CAD build for the part. Positions are in the model's coordinates, mm. Face numbers are marked on the shaded views. A direction names the side the tool comes from. Round coordinates to 2 decimals unless told otherwise and drop trailing zeros. Order: outer loops, then holes, each group sorted by start corner. A loop starts at its lowest first (then second) coordinate and runs counter-clockwise, first axis right, second up. Notation, with made-up numbers: M -4.5,9.25 L 52.5,9.25 A32 ccw 52.5,36.25 Z; hole C 47,27 d10. An arc over 180 degrees is marked long. Answer as a JSON object with one key per item and string values.
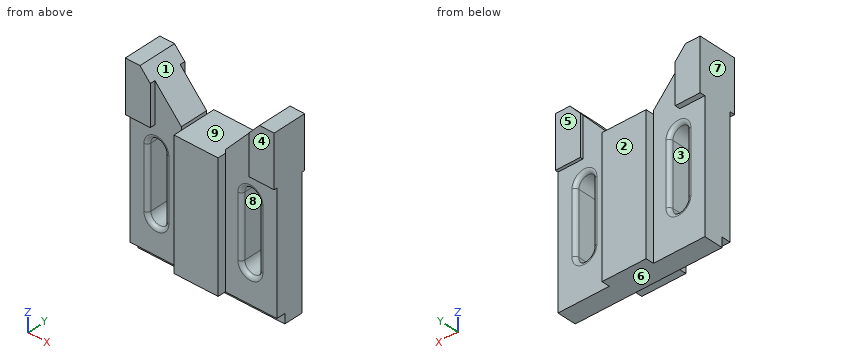
```python
from build123d import *

# Parameters (mm, degrees)
F1_DEPTH  = 15
F3_W      = 11.5
F3_H      = 6.5
F4_DEPTH  = 100
F6_DEPTH  = 5.5
F8_DEPTH  = 3.5
F10_DEPTH = 5.5
F12_DEPTH = 3.5
F14_DEPTH = 25
F15_R     = 2.5
F16_W     = 20.5905072875
F16_H     = 35
F16_W_2   = 2
F17_DEPTH = 17


with BuildPart() as f1:
    # F0 (on Front) → F1 (new body, symmetric)
    with BuildSketch(Plane.XZ):
        Polygon((0, 122), (0, 0), (100, 0), (100, 122), (90, 122), (65, 94.2346871293), (65, 92), (35, 92), (35, 94.2346871293), (10, 122), align=None)
    extrude(amount=F1_DEPTH, both=True)

    # F3 (on face) → F4 (cut)
    with BuildSketch(Plane(origin=(0, 0, 0), x_dir=(0, -1, 0), z_dir=(-1, 0, 0))):
        with Locations((9.25, 3.25)):
            Rectangle(F3_W, F3_H)
    extrude(amount=-F4_DEPTH, mode=Mode.SUBTRACT)

    # F5 (on face) → F6 (cut)
    with BuildSketch(Plane.XZ.offset(15)):
        Polygon((17, 87), (0, 87), (0, 6.5), (35, 6.5), (35, 92), (35, 94.2346871293), (17, 114.2257123962), align=None)
        Polygon((65, 94.2346871293), (65, 92), (65, 6.5), (100, 6.5), (100, 87), (83, 87), (83, 114.2257123962), align=None)
    extrude(amount=-F6_DEPTH, mode=Mode.SUBTRACT)

    # F7 (on face) → F8 (cut)
    with BuildSketch(Plane.XZ.offset(15)):
        Polygon((100, 122), (90, 122), (83, 114.2257123962), (83, 87), (100, 87), align=None)
    extrude(amount=-F8_DEPTH, mode=Mode.SUBTRACT)

    # F9 (on face) → F10 (cut)
    with BuildSketch(Plane(origin=(0, 15, 0), x_dir=(-1, 0, 0), z_dir=(0, 1, 0))):
        Polygon((-17, 87), (-17, 114.2257123962), (-35, 94.2346871293), (-35, 92), (-35, 0), (0, 0), (0, 87), align=None)
        Polygon((-65, 92), (-65, 94.2346871293), (-83, 114.2257123962), (-83, 87), (-100, 87), (-100, 0), (-65, 0), align=None)
    extrude(amount=-F10_DEPTH, mode=Mode.SUBTRACT)

    # F11 (on face) → F12 (cut)
    with BuildSketch(Plane(origin=(0, 15, 0), x_dir=(-1, 0, 0), z_dir=(0, 1, 0))):
        Polygon((-90, 122), (-100, 122), (-100, 87), (-83, 87), (-83, 114.2257123962), align=None)
    extrude(amount=-F12_DEPTH, mode=Mode.SUBTRACT)

    # F13 (on face) → F14 (cut)
    with BuildSketch(Plane.XZ.offset(15)):
        with BuildLine():
            Line((24, 30), (24, 72))
            ThreePointArc((24, 72), (18, 78), (12, 72))
            Line((12, 72), (12, 30))
            ThreePointArc((12, 30), (18, 24), (24, 30))
        make_face()
        with BuildLine():
            ThreePointArc((88, 72), (82, 78), (76, 72))
            Line((76, 72), (76, 30))
            ThreePointArc((76, 30), (82, 24), (88, 30))
            Line((88, 30), (88, 72))
        make_face()
    extrude(amount=-F14_DEPTH, mode=Mode.SUBTRACT)

    # F15
    f15_edges = [f1.edges().sort_by_distance(p)[0] for p in [
        (76, 9.5, 51),
        (24, 9.5, 51),
        (12, -9.5, 51),
        (76, -9.5, 51),
    ]]
    fillet(f15_edges, radius=F15_R)

    # F16 (on face) → F17 (cut)
    with BuildSketch(Plane(origin=(0, 0, 0), x_dir=(0, -1, 0), z_dir=(-1, 0, 0))):
        with Locations((-25.2952536438, 104.5)):
            Rectangle(F16_W, F16_H)
        with Locations((25.2952536438, 104.5)):
            Rectangle(F16_W, F16_H)
        with Locations((-14, 104.5)):
            Rectangle(F16_W_2, F16_H)
        with Locations((14, 104.5)):
            Rectangle(F16_W_2, F16_H)
    extrude(amount=-F17_DEPTH, mode=Mode.SUBTRACT)


solid = f1.part
```
Item 1: Saw through at D-D on z = 109. List the corners of the cut face in (x, y), and give its area (3 significant figures).
Worked answers:
{"outline": "M 0,-13 L 17,-13 L 17,-9.5 L 21.71,-9.5 L 21.71,9.5 L 17,9.5 L 17,13 L 0,13 Z; M 78.29,-9.5 L 83,-9.5 L 83,-11.5 L 100,-11.5 L 100,11.5 L 83,11.5 L 83,9.5 L 78.29,9.5 Z", "area": "1,010 mm2"}
Item 2: Saw through at A-A on y = 3.75. List the corners of the cut face in (x, z), and give its area (3 significant figures).
Worked answers:
{"outline": "M 0,0 L 100,0 L 100,122 L 90,122 L 65,94.23 L 65,92 L 35,92 L 35,94.23 L 10,122 L 0,122 Z; hole M 12,30 A6 ccw 24,30 L 24,72 A6 ccw 12,72 Z; hole M 76,30 A6 ccw 88,30 L 88,72 A6 ccw 76,72 Z", "area": "9,370 mm2"}
Item 3: Saw through at C-C on x = 49. List the corners of the cut face in (y, z).
Worked answers:
{"outline": "M -15,6.5 L -3.5,6.5 L -3.5,0 L 15,0 L 15,92 L -15,92 Z"}
Item 4: Saw through at B-B on z = 64. List the corners of the cut face in (x, y).
Worked answers:
{"outline": "M 0,-9.5 L 9.5,-9.5 A2.5 ccw 12,-7 L 12,7 A2.5 ccw 9.5,9.5 L 0,9.5 Z; M 24,-7 A2.5 ccw 26.5,-9.5 L 35,-9.5 L 35,-15 L 65,-15 L 65,-9.5 L 73.5,-9.5 A2.5 ccw 76,-7 L 76,7 A2.5 ccw 73.5,9.5 L 65,9.5 L 65,15 L 35,15 L 35,9.5 L 26.5,9.5 A2.5 ccw 24,7 Z; M 88,-7 A2.5 ccw 90.5,-9.5 L 100,-9.5 L 100,9.5 L 90.5,9.5 A2.5 ccw 88,7 Z"}
Item 5: 3-axis set-ups, long thin cutter, end or side, ignore diameter. For the marked faces 1, 2, 3, 4 and 5: which of +Z, -Z, +X, -X, +Y, -Y reach the whole face in a straight line?
Worked answers:
{"face 1": "+Z, +Y, -Y", "face 2": "+Z, -Z, +X, -X, +Y", "face 3": "+Y, -Y", "face 4": "+Z, -Z, +X, -Y", "face 5": "+Z, -Z, +X, +Y"}
Item 6: Wall check: line 1 along X through (y, z) = (2.5, 30); line 2 along X through (y, z) = (-12.5, 76); line 3 along Y through (x, z) = (7, 106). Give the ranges that are in metal, low to high. Write a range as [from, to].
Worked answers:
{"line 1": "x = [0, 12], [24, 76], [88, 100]", "line 2": "x = [35, 65]", "line 3": "y = [-13, 13]"}
Item 7: Drop flat-ended pins along their axis: pin 1 Ø3 at (y, z) = (-12.5, 64) entering from -X; pin 2 Ø17.5 at (x, z) = (85.5, 52) entering from +Y; pin 3 Ø3 at (x, y) = (38, 11) entering from +Z. Give the stop position or say it passes through.
Worked answers:
{"pin 1": "stops at x = 35", "pin 2": "stops at y = 9.5", "pin 3": "stops at z = 92"}
Item 8: Two-plate mould, pull along X, no slides. Class the marked faces 6, 7, 8 and 9: released by +X, released by -X, zero draft, split by the parting line, or undercut.
Worked answers:
{"face 6": "zero draft", "face 7": "released by -X", "face 8": "undercut", "face 9": "undercut"}
